from build123d import *

# Parameters (mm, degrees)
F0_W     = 55.539488
F0_H     = 32.094934
F1_DEPTH = 25
F3_DEPTH = 10
F4_DEPTH = 10


with BuildPart() as f1:
    # F0 (on Top) → F1 (new body)
    with BuildSketch(Plane.XY):
        Rectangle(F0_W, F0_H)
    extrude(amount=-F1_DEPTH)

    # F2 (on face) → F3 (cut)
    with BuildSketch(Plane.XY):
        with BuildLine():
            ThreePointArc((0, 5.113803), (-5, 0.113803), (0, -4.886197))
            Line((0, -4.886197), (0, 5.113803))
        make_face()
    extrude(amount=-F3_DEPTH, mode=Mode.SUBTRACT)

    # F2 (on face) → F4 (cut)
    with BuildSketch(Plane.XY):
        with BuildLine():
            Line((0, 5.113803), (0, -4.886197))
            ThreePointArc((0, -4.886197), (5, 0.113803), (0, 5.113803))
        make_face()
    extrude(amount=-F4_DEPTH, mode=Mode.SUBTRACT)


solid = f1.part
Read the model definition and answer for the solid it produces. Units are mm, in the model's axes. A direction names the side the tool comes from. Give positions to 0.01 mm unless a question says otherwise; leave off trailing zeros. Write each loop counter-clockwise with the first axis right and the second up, starting at its lowest first coordinate (ties: lowest second). Pieces come first, ordered by that corner, then holes. Notation, with made-up numbers: (49, -25) - (87, -25) arc R13 ccw to (87, -16) - close; hole circle Ø7 at (22, -7.75). An arc over 180 degrees is marked (long way). Use CSV: the item, a comma, the result in double quotes. Start each with the question number.
(1) Find section C-C (y = -3). Give the vertices of the cut face in (x, z).
(2) Determine the mould class of faces 1 (the flat face through (0, -16.047, -12)), 2 (the flat face through (-27.77, 0, -12)), 3 (the flat face through (0, 0, -10)) for opening direction X: +X half, -X half, draft (parallel to the pull), parting line (faces both ways), or undercut.
(3) For faces 4 (the cylindrical face through (4.88, -0.97, -4.93)), 5 (the flat face through (-7, 0, 0)), determine the directions among +Z, -Z, +X, -X, +Y, -Y from which every point of the face is accessible in a straight line to the end or side of a thin tool.
(4) Consider line 1 along X through (y, z) = (1.5, -5.75). Determine where the line is inside the solid, lowest interval first.
(5) Find section B-B (z = -2.75). Give the vertices of the cut face in (x, y).
(6) Find section A-A (x = 0). Give the vertices of the cut face in (y, z).
Findings below:
1,outline,"(-27.77, -25) - (27.77, -25) - (27.77, 0) - (3.91, 0) - (3.91, -10) - (-3.91, -10) - (-3.91, 0) - (-27.77, 0) - close"
2,face 1,"draft"
2,face 2,"-X half"
2,face 3,"undercut"
3,face 4,"+Z"
3,face 5,"+Z, +X, -X, +Y, -Y"
4,line 1,"-27.77 to -4.8, 4.8 to 27.77"
5,outline,"(-27.77, -16.05) - (27.77, -16.05) - (27.77, 16.05) - (-27.77, 16.05) - close; hole circle Ø10 at (0, 0.11)"
6,outline,"(-16.05, -25) - (16.05, -25) - (16.05, 0) - (5.11, 0) - (5.11, -10) - (-4.89, -10) - (-4.89, 0) - (-16.05, 0) - close"
